Source: three-view drawing plus pictorial views. Frame: mm from the lowest corner of the part. A direction names the side the tool comes from. Coordinates: 2 decimals unless noted, no trailing zeros. Loops run counter-clockwise (first coordinate to the right, second up) from the corner with the lowest first, then second, coordinate; pieces in that order, holes last. Notation, with made-up numbers: M -20,-24.75 L 32,-24.75 A26 ccw 32,1.25 Z; hole C -28.5,0 d1. An arc over 180 degrees is marked long. Use a Markdown table: item, result. Add a question column.
1. Section C-C on x = 24.75. Output: boundary loops of the cut face in (y, z) (1 decimal).
2. Set-up query: the marked faces 3, 4 and 5. Return all of +Z, -Z, +X, -X, +Y, -Y with unobstructed straight access to the full face (end or side cutting, diameter ignored); none if empty.
3. Section D-D on z = 4. Output: boundary loops of the cut face in (x, y) (1 decimal).
4. Section B-B on x = 14.75. Output: boundary loops of the cut face in (y, z) (1 decimal).
5. Line query: L1, parallel to Y at x = 5.75, z = 23.75; L2, parallel to Z at x = 17, y = 17.5 (1 decimal); L3, parallel to X at y = 29.5, z = 18 (1 decimal). Output: solid intervals per line, ascending. Write a range as [from, to].
6. Draft query along X for the marked faces 1 and 2. Return one class per face: +X half, -X half, draft (parallel to the pull), parting line (faces both ways), or undercut.
7. Section A-A on z = 20.5. Output: boundary loops of the cut face in (x, y) (1 decimal), then the cut area to 3 significant figures.
8. Pin query (flat end, axial travel): pin 1 (3 mm diameter, centred on y = 17, z = 23, fed in from -X); pin 2 (12 mm diameter, centred on y = 23, z = 6, fed in from -X); pin 3 (5 mm diameter, centred on x = 12.5, y = 17.5, fed in from -Z). Return the tip coordinate at first contact, or that it passes through.
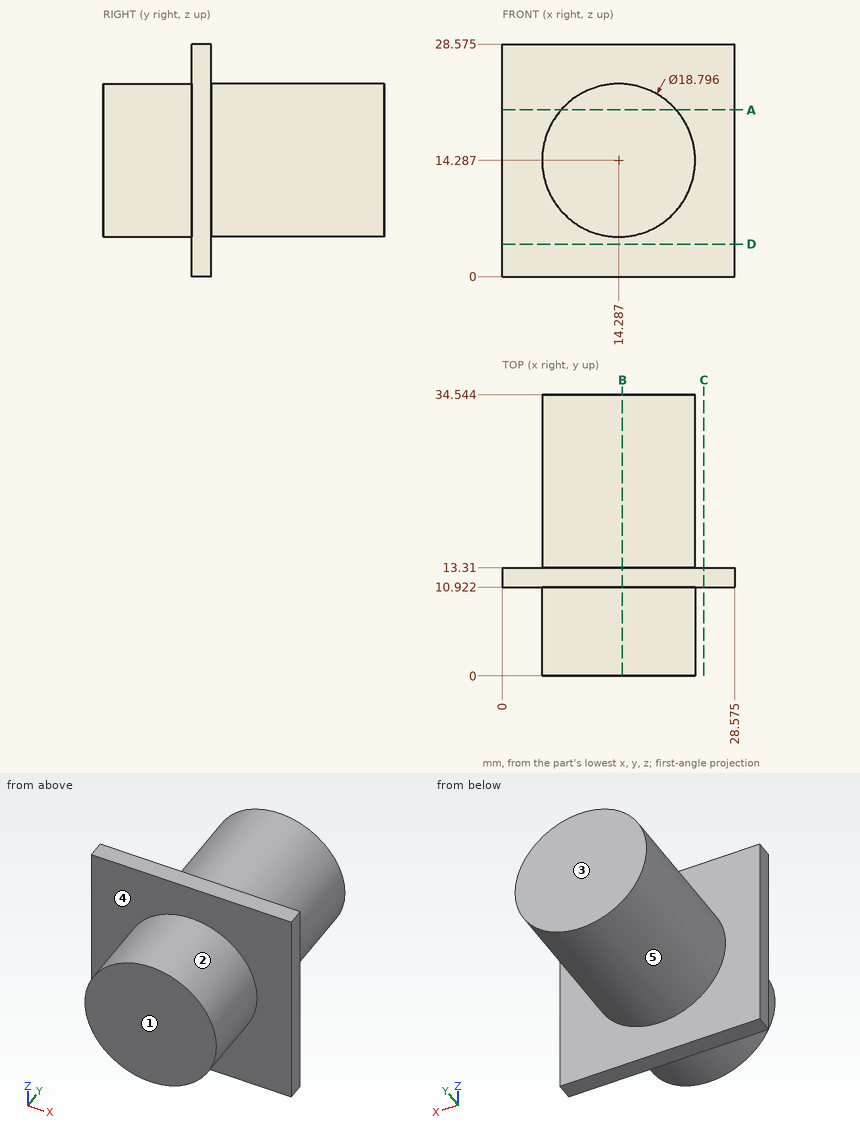
Answers below:
| question | item | result |
|---|---|---|
| 1 | outline | M 10.9,0 L 13.3,0 L 13.3,28.6 L 10.9,28.6 Z |
| 2 | face 3 | +Z, -Z, +X, -X, +Y |
| 2 | face 4 | -Y |
| 2 | face 5 | +Y |
| 3 | outline | M 0,10.9 L 28.6,10.9 L 28.6,13.3 L 0,13.3 Z |
| 4 | outline | M 0,4.9 L 10.9,4.9 L 10.9,0 L 13.3,0 L 13.3,4.9 L 34.5,4.9 L 34.5,23.7 L 13.3,23.7 L 13.3,28.6 L 10.9,28.6 L 10.9,23.7 L 0,23.7 Z |
| 5 | L1 | y = [10.92, 13.31] |
| 5 | L2 | z = [5.3, 23.3] |
| 5 | L3 | x = [5.7, 22.9] |
| 6 | face 1 | draft |
| 6 | face 2 | parting line |
| 7 | outline | M 0,10.9 L 7.2,10.9 L 7.2,0 L 21.3,0 L 21.3,10.9 L 28.6,10.9 L 28.6,13.3 L 21.3,13.3 L 21.3,34.5 L 7.2,34.5 L 7.2,13.3 L 0,13.3 Z |
| 7 | area | 522 mm² |
| 8 | pin 1 | stops at x = 8.26 |
| 8 | pin 2 | stops at x = 5.17 |
| 8 | pin 3 | stops at z = 4.89 |
